Autodesk Inventor part; units mm, degrees
ref_plane "YZ Plane" through (0, 0, 0) normal (1, 0, 0) x (0, 1, 0)
ref_plane "XZ Plane" through (0, 0, 0) normal (0, 1, 0) x (-1, 0, 0)
ref_plane "XY Plane" through (0, 0, 0) normal (0, 0, 1) x (1, 0, 0)
sketch "草图1" plane through (0, 0, 0) normal (0, 0, 1) x (1, 0, 0)
  line L0 (150, -100) -> (-150, -100)
  line L1 (-150, -100) -> (-150, 100)
  line L2 (-150, 100) -> (150, 100)
  line L3 (150, 100) -> (150, -100)
  line L4 (150, -100) -> (-150, 100) construction
  line L5 (-150, -100) -> (150, 100) construction
  point P0 (0, 0)
  dimension "d0" = 300
  dimension "d1" = 200
extrude "拉伸1" add sketch "草图1" along normal mid plane 20
sketch "草图2" plane through (0, 0, 10) normal (0, 0, 1) x (1, 0, 0)
  line L0 (150, 100) -> (-150, 100) construction
  line L1 (-150, 100) -> (-150, -100) construction
  line L2 (-150, -100) -> (150, -100) construction
  line L3 (150, -100) -> (150, 100) construction
  line L4 (150, 100) -> (-150, 100) construction
  circle A0 centre (-87.5, 100) radius 20
  line L5 (0, 0) -> (0, 160.0465) construction
  circle A1 centre (87.5, 100) radius 20
  dimension "d4" = 40
  dimension "d5" = 175
extrude "拉伸2" cut sketch "草图2" against normal blind 20
sketch "草图3" plane through (-150, -100, 10) normal (0, -1, 0) x (1, 0, 0)
  line L0 (300, -20) -> (300, 0) construction
  line L1 (0, 0) -> (300, 0) construction
  line L2 (0, -20) -> (0, 0) construction
  line L3 (300, -20) -> (0, -20) construction
  line L4 (0, -20) -> (42.5, -20)
  line L5 (150, -10) -> (150, 57.6375)
  line L6 (300, -20) -> (300, 0) construction
  line L7 (300, -20) -> (257.5, -20) construction
  line L8 (0, 0) -> (300, 0)
  line L9 (40, 0) -> (60, 0)
  line L10 (60, 0) -> (60, -50)
  line L11 (60, -50) -> (40, -50)
  line L12 (40, -50) -> (40, 0)
  line L13 (300, -20) -> (300, 0) construction
  line L14 (300, -20) -> (257.5, -20)
  line L15 (260, 0) -> (240, 0)
  line L16 (240, 0) -> (240, -50)
  line L17 (240, -50) -> (260, -50)
  line L18 (260, -50) -> (260, 0)
  point P0 (260, 0)
  point P1 (240, 0)
  dimension "d20" = 20
  dimension "d21" = 50
  dimension "d22" = 180
extrude "拉伸4" add sketch "草图3" against normal blind 10
full round fillet "全圆角3" first side at (110, -96.6667, -30) centre faces at (96.6667, -96.6667, -40) second side at (90, -96.6667, -20)
mirror "镜像1" about plane through (0, 0, 0) normal (1, 0, 0) of "全圆角3"
sketch "草图5" plane through (-150, -90, 10) normal (0, 1, 0) x (1, 0, 0)
  arc A0 (260, 40) -> (240, 40) centre (250, 40) ccw
  arc A1 (60, 40) -> (40, 40) centre (50, 40) ccw
  point P0 (150, 10)
hole "孔2" at (100, -90, -30) at (-100, -90, -30) direction (0, -1, 0) diameter 10 end through all
properties part number "支撑板1"
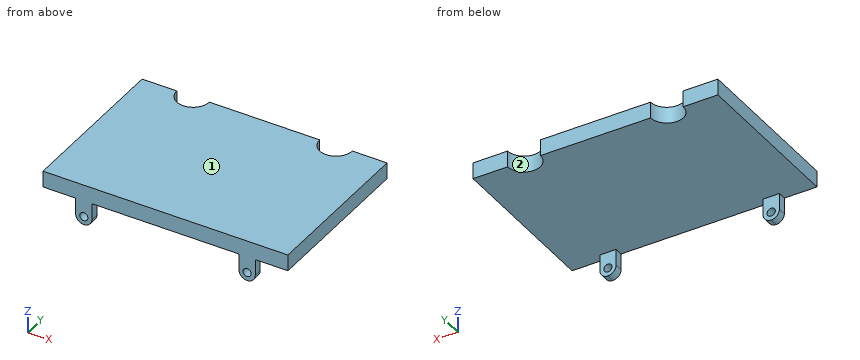
Geometry check sheet. Reference: the model listing, model coordinates, mm. Face numbers are marked on the shaded views. Coordinates: 2 decimals unless noted, no trailing zeros. Order: outer loops, then holes, each group sorted by start corner. A loop starts at its lowest first (then second) coordinate and runs counter-clockwise, first axis right, second up.
Q1. Depth check by flat-ended pin: pin 1 Ø3 at (x, y) = (-79, -63.5) entering from -Z; pin 2 Ø5 at (y, z) = (-96.5, -16) entering from -X; pin 3 Ø8 at (x, z) = (92.5, -13.5) entering from +Y; pin 4 Ø6 at (x, z) = (100, -30) entering from -Y. Enter the tip coordinate at first touch or a pass-through.
Reply:
pin 1: stops at z = -10
pin 2: stops at x = -110
pin 3: stops at y = 81.24
pin 4: passes through
Q2. Sectioned sample at A-A on z = -2. Record the cut outline in (x, y).
Reply:
outline: (-150, -100) - (150, -100) - (150, 100) - (107.5, 100) arc R20 cw to (67.5, 100) - (-67.5, 100) arc R20 cw to (-107.5, 100) - (-150, 100) - close
Q3. Thickness scan on probe 1 along X at (y, z) = (-97, -30); probe 2 along Z at (x, y) = (100, -94); probe 3 along Y at (x, z) = (-106.5, -31). Record the ranges inside material, lowest first.
Reply:
probe 1: x = -110 to -105, -95 to -90, 90 to 95, 105 to 110
probe 2: z = -40 to -35, -25 to 10
probe 3: y = -100 to -90
Q4. Sectioned sample at C-C on x = -25.5. Record the cut outline in (y, z), and give its area (3 significant figures).
Reply:
outline: (-100, -10) - (100, -10) - (100, 10) - (-100, 10) - close
area: 4,000 mm2
Q5. Draft check along X on the marked faces 1 and 2. Enter one of: released by +X, released by -X, zero draft, split by the parting line, or undercut.
Reply:
face 1: zero draft
face 2: undercut
Q6. Sectioned sample at B-B on y = 4. Record the cut outline in (x, z), and give its area (3 significant figures).
Reply:
outline: (-150, -10) - (150, -10) - (150, 10) - (-150, 10) - close
area: 6,000 mm2
